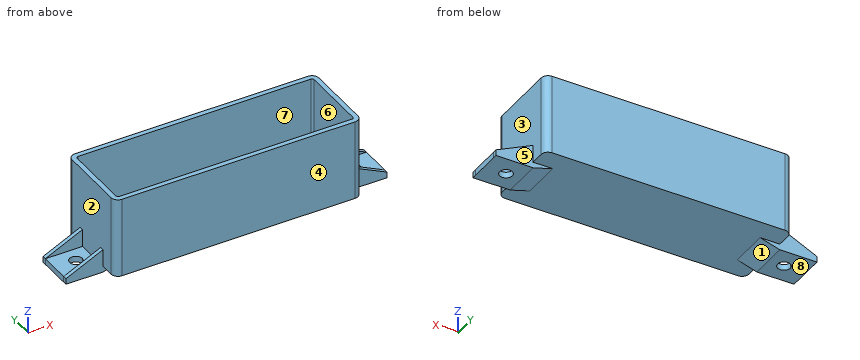
```python
from build123d import *

# Parameters (mm, degrees)
F0_W     = 126
F0_H     = 41
F0_W_2   = 121
F0_H_2   = 36
F1_DEPTH = 41
F2_DEPTH = 3
F3_W     = 10
F3_H     = 2
F3_H_2   = 16
F4_DEPTH = 3
F5_DEPTH = 3
F6_DEPTH = 6
F8_DEPTH = 20
F9_R     = 3.5
F10_R    = 1


with BuildPart() as f1:
    # F0 (on Top) → F1 (new body)
    with BuildSketch(Plane.XY):
        Rectangle(F0_W, F0_H)
        Rectangle(F0_W_2, F0_H_2, mode=Mode.SUBTRACT)
    extrude(amount=F1_DEPTH)

    # F0 (on Top) → F2 (join)
    with BuildSketch(Plane.XY):
        Rectangle(F0_W_2, F0_H_2)
    extrude(amount=F2_DEPTH)

    # F3 (on Top) → F4 (join, symmetric)
    with BuildSketch(Plane.XY):
        Polygon((-82, 8), (-81.9793343544, 8), (-63, 8), (-63, 10), (-82, 10), align=None)
        with Locations((-58, 9)):
            Rectangle(F3_W, F3_H)
        with Locations((-58, 0)):
            Rectangle(F3_W, F3_H_2)
        Polygon((-63, -10), (-63, -8), (-81.9793343544, -8), (-82, -10), align=None)
        with Locations((-58, -9)):
            Rectangle(F3_W, F3_H)
        Polygon((81.9793343544, -8), (63, -8), (63, -10), (82, -10), align=None)
        with Locations((58, -9)):
            Rectangle(F3_W, F3_H)
        with Locations((58, 0)):
            Rectangle(F3_W, F3_H_2)
        with Locations((58, 9)):
            Rectangle(F3_W, F3_H)
        Polygon((63, 8), (81.9793343544, 8), (82, 8), (82, 10), (63, 10), align=None)
    extrude(amount=F4_DEPTH, both=True)

    # F3 (on Top) → F5 (join)
    with BuildSketch(Plane.XY):
        Polygon((82, 8), (81.9793343544, 8), (63, 8), (63, -8), (81.9793343544, -8), (81.9896671772, 0), align=None)
        with BuildLine():
            ThreePointArc((74.2396763525, 0.0142076195), (74.2396756748, 0.0121087662), (74.2396736416, 0.0100099137))
            ThreePointArc((74.2396736416, 0.0100099137), (67.7396770302, 0.0163064728), (74.2396763525, 0.0142076195))
        make_face(mode=Mode.SUBTRACT)
        Polygon((-63, 8), (-81.9793343544, 8), (-82, 8), (-81.9896671772, 0), (-81.9793343544, -8), (-63, -8), align=None)
        with BuildLine():
            ThreePointArc((-67.7396763525, 0.0142076195), (-70.9875774992, -3.2357917028), (-74.2396736416, 0.0100099137))
            ThreePointArc((-74.2396736416, 0.0100099137), (-70.9917752058, 3.2642069418), (-67.7396763525, 0.0142076195))
        make_face(mode=Mode.SUBTRACT)
    extrude(amount=-F5_DEPTH)

    # F6 (add): faces of the model
    f6_faces = [f1.faces().sort_by_distance(p)[0] for p in [
        (-72.5, 9, 3),
        (-72.4948345257, -9.0001813762, 3),
        (72.5, 9, 3),
        (72.4948345257, -9.0001813762, 3),
    ]]
    extrude(f6_faces, amount=F6_DEPTH)

    # F7 (on face) → F8 (cut)
    with BuildSketch(Plane.XZ.offset(10)):
        Polygon((63, 9), (82, 0), (82, 9), align=None)
        Polygon((53, -3), (63, -3), (53, 0), align=None)
        Polygon((-82, 9), (-82, 0), (-63, 9), align=None)
        Polygon((-53, 0), (-63, -3), (-53, -3), align=None)
    extrude(amount=-F8_DEPTH, mode=Mode.SUBTRACT)

    # F9
    f9_edges = [f1.edges().sort_by_distance(p)[0] for p in [
        (-63, -20.5, 20.5),
        (-63, 20.5, 20.5),
        (63, 20.5, 20.5),
        (63, -20.5, 20.5),
    ]]
    fillet(f9_edges, radius=F9_R)

    # F10
    f10_edges = [f1.edges().sort_by_distance(p)[0] for p in [
        (0, -18, 3),
        (60.5, 0, 3),
        (60.5, -18, 22),
        (0, 18, 3),
        (60.5, 18, 22),
        (-60.5, 0, 3),
        (-60.5, 18, 22),
        (-60.5, -18, 22),
    ]]
    fillet(f10_edges, radius=F10_R)


solid = f1.part
```
Input: part model. Units: mm. Frame: model coordinates. Face numbers are marked on the shaded views. A direction names the side the tool comes from. Coordinates: 2 decimals unless noted, no trailing zeros. Loops run counter-clockwise (first coordinate to the right, second up) from the corner with the lowest first, then second, coordinate; pieces in that order, holes last. Notation, with made-up numbers: M 84.5,19.5 L 127.5,19.5 A31 ccw 127.5,58.5 Z; hole C 10.5,-27 d4. An arc over 180 degrees is marked long. One line per item, written item: value.
(1) Section B-B (x = 22). Output: boundary loops of the cut face in (y, z).
Filled in:
outline: M -20.5,0 L 20.5,0 L 20.5,41 L 18,41 L 18,4 A1 cw 17,3 L -17,3 A1 cw -18,4 L -18,41 L -20.5,41 Z
(2) Section A-A (z = 14). Output: boundary loops of the cut face in (x, y), and give its area (3 significant figures).
Filled in:
outline: M -63,-17 A3.5 ccw -59.5,-20.5 L 59.5,-20.5 A3.5 ccw 63,-17 L 63,17 A3.5 ccw 59.5,20.5 L -59.5,20.5 A3.5 ccw -63,17 Z; hole M -60.5,-17 A1 ccw -59.5,-18 L 59.5,-18 A1 ccw 60.5,-17 L 60.5,17 A1 ccw 59.5,18 L -59.5,18 A1 ccw -60.5,17 Z
area: 800 mm^2
(3) Reachability of the marked faces 1, 2, 3 and 4 from +Z, -Z, +X, -X, +Y, -Y: full face, straight path, thin tool, end or side. Return the list, or none.
Filled in:
face 1: -Z, +Y, -Y
face 2: +Z, -X
face 3: +Z, +X
face 4: +Z, -Z, +X, -X, -Y
(4) Pin query (flat end, axial travel): pin 1 (10 mm diameter, centred on y = 8, z = 3.5, fed in from -X); pin 2 (7 mm diameter, centred on x = -70, z = 4.5, fed in from +Y); pin 3 (2.5 mm diameter, centred on x = 76, z = 4.5, fed in from +Y); pin 4 (6 mm diameter, centred on x = -63, z = 6, fed in from -Y). Return the tip coordinate at first contact, or that it passes through.
Filled in:
pin 1: x = -82
pin 2: y = 10
pin 3: through
pin 4: y = -20.46
(5) Section C-C (y = 15.5). Output: boundary loops of the cut face in (x, z).
Filled in:
outline: M -63,0 L 63,0 L 63,41 L 60.5,41 L 60.5,4 A1 cw 59.5,3 L -59.5,3 A1 cw -60.5,4 L -60.5,41 L -63,41 Z
(6) Pull-direction query (Y, two-part tool) for the marked faces 5, 6, 7 and 8; classes: +Y half, -Y half, draft (parallel to the pull), parting line (faces both ways), or undercut.
Filled in:
face 5: +Y half
face 6: undercut
face 7: undercut
face 8: draft
(7) Line query: line 1 along Y through (x, z) = (41, 27.5); line 2 along X through (y, z) = (-2, 30); line 3 along Z through (x, y) = (20, -7). Output: solid intervals per line, ascending. Write a range as from..to.
Filled in:
line 1: -20.5..-18, 18..20.5
line 2: -63..-60.5, 60.5..63
line 3: 0..3
